Read the model definition and answer for the solid it produces. Units are mm, in the model's axes. A direction names the side the tool comes from. Coordinates: 2 decimals unless noted, no trailing zeros. Loops run counter-clockwise (first coordinate to the right, second up) from the corner with the lowest first, then second, coordinate; pieces in that order, holes last.
from build123d import *

# Parameters (mm, degrees)
SKETCH1_W                      = 120
SKETCH1_H                      = 200
BASE_FLANGE1_DEPTH             = 1.2
EDGE_FLANGE1_STRIP_W           = 6.2732
EDGE_FLANGE1_STRIP_H           = 1.2
EDGE_FLANGE1_STRIP_CUT_DEPTH   = 120
EDGE_FLANGE1_STRIP_2_W         = 6.2732
EDGE_FLANGE1_STRIP_2_H         = 1.2
EDGE_FLANGE1_STRIP_CUT_2_DEPTH = 120
EDGE_FLANGE1_DEPTH             = 120
EDGE_FLANGE1_BEND_DEPTH        = 120
EDGE_FLANGE3_START             = -121.9366
EDGE_FLANGE3_OUTLINE_W         = 50
EDGE_FLANGE3_OUTLINE_H         = 1.2
EDGE_FLANGE3_DEPTH             = 123.8732
EDGE_FLANGE3_START_2           = -25
EDGE_FLANGE3_2_DEPTH           = 50
EDGE_FLANGE3_START_3           = -65
EDGE_FLANGE3_3_DEPTH           = 130
EDGE_FLANGE4_STRIP_W           = 6.2732
EDGE_FLANGE4_STRIP_H           = 1.2
EDGE_FLANGE4_STRIP_CUT_DEPTH   = 120
EDGE_FLANGE4_STRIP_2_W         = 6.2732
EDGE_FLANGE4_STRIP_2_H         = 1.2
EDGE_FLANGE4_STRIP_CUT_2_DEPTH = 120
EDGE_FLANGE4_DEPTH             = 120
EDGE_FLANGE4_BEND_DEPTH        = 120
SKETCH34_R                     = 4
CUT_EXTRUDE1_DEPTH             = 10
CUT_EXTRUDE2_DEPTH             = 10
SKETCH36_R                     = 2.5
CUT_EXTRUDE3_DEPTH             = 243.320330787
SKETCH37_R                     = 2.5
CUT_EXTRUDE4_DEPTH             = 10


with BuildPart() as part:
    # Base-Flange1: sheet metal written as solids
    # Sketch1 → Base-Flange1 (new body)
    with BuildSketch(Plane.XY):
        Rectangle(SKETCH1_W, SKETCH1_H)
    extrude(amount=-BASE_FLANGE1_DEPTH)

    # Edge-Flange1: sheet metal written as solids
    # Edge-Flange1 strip (on a plane across the edge) → Edge-Flange1 strip cut (cut)
    with BuildSketch(Plane(origin=(-60, 100, -1.2), x_dir=(0, -1, 0), z_dir=(1, 0, 0))):
        with Locations((-1.2, -0.6)):
            Rectangle(EDGE_FLANGE1_STRIP_W, EDGE_FLANGE1_STRIP_H)
    extrude(amount=EDGE_FLANGE1_STRIP_CUT_DEPTH, mode=Mode.SUBTRACT)

    # Edge-Flange1 strip 2 (on a plane across the edge) → Edge-Flange1 strip cut 2 (cut)
    with BuildSketch(Plane(origin=(60, -100, -1.2), x_dir=(0, 1, 0), z_dir=(-1, 0, 0))):
        with Locations((-1.2, -0.6)):
            Rectangle(EDGE_FLANGE1_STRIP_2_W, EDGE_FLANGE1_STRIP_2_H)
    extrude(amount=EDGE_FLANGE1_STRIP_CUT_2_DEPTH, mode=Mode.SUBTRACT)

    # Edge-Flange1 section (on a plane across the edge) → Edge-Flange1 (add)
    with BuildSketch(Plane(origin=(-60, 100, -1.2), x_dir=(0, -1, 0), z_dir=(1, 0, 0))):
        with BuildLine():
            Line((0, 0.7366), (0, 178.8))
            Line((0, 178.8), (1.2, 178.8))
            Line((1.2, 178.8), (1.2, 0.7366))
            ThreePointArc((1.2, 0.7366), (1.415745145, 0.215745145), (1.9366, 0))
            Line((1.9366, 0), (1.9366, -1.2))
            ThreePointArc((1.9366, -1.2), (0.567217008, -0.632782992), (0, 0.7366))
        make_face()
    extrude(amount=EDGE_FLANGE1_DEPTH)

    # Edge-Flange1 section 2 (on a plane across the edge) → Edge-Flange1 bend (add)
    with BuildSketch(Plane(origin=(60, -100, -1.2), x_dir=(0, 1, 0), z_dir=(-1, 0, 0))):
        with BuildLine():
            Line((0, 0.7366), (0, 178.8))
            Line((0, 178.8), (1.2, 178.8))
            Line((1.2, 178.8), (1.2, 0.7366))
            ThreePointArc((1.2, 0.7366), (1.415745145, 0.215745145), (1.9366, 0))
            Line((1.9366, 0), (1.9366, -1.2))
            ThreePointArc((1.9366, -1.2), (0.567217008, -0.632782992), (0, 0.7366))
        make_face()
    extrude(amount=EDGE_FLANGE1_BEND_DEPTH)

    # Edge-Flange3: read off the stored shape, not the designer's step
    # Edge-Flange3 outline → Edge-Flange3 (add)
    with BuildSketch(Plane(origin=(60, 0, -1.2), x_dir=(0, -1, 0), z_dir=(1, 0, 0)).offset(EDGE_FLANGE3_START)):
        with Locations((0, -0.6)):
            Rectangle(EDGE_FLANGE3_OUTLINE_W, EDGE_FLANGE3_OUTLINE_H)
    extrude(amount=EDGE_FLANGE3_DEPTH)

    # Edge-Flange3 2 outline → Edge-Flange3 2 (add)
    with BuildSketch(Plane(origin=(0, 0, 0), x_dir=(1, 0, 0), z_dir=(0, 1, 0)).offset(EDGE_FLANGE3_START_2)):
        with BuildLine():
            ThreePointArc((61.9366, 0), (63.305982992, 0.567217008), (63.8732, 1.9366))
            Line((63.8732, 1.9366), (63.8732, 31.2))
            Line((63.8732, 31.2), (62.6732, 31.2))
            Line((62.6732, 31.2), (62.6732, 1.9366))
            ThreePointArc((62.6732, 1.9366), (62.457454855, 1.415745145), (61.9366, 1.2))
            Line((61.9366, 1.2), (61.9366, 0))
        make_face()
        with BuildLine():
            Line((-62.6732, 31.2), (-63.8732, 31.2))
            Line((-63.8732, 31.2), (-63.8732, 1.9366))
            ThreePointArc((-63.8732, 1.9366), (-63.305982992, 0.567217008), (-61.9366, 0))
            Line((-61.9366, 0), (-61.9366, 1.2))
            ThreePointArc((-61.9366, 1.2), (-62.457454855, 1.415745145), (-62.6732, 1.9366))
            Line((-62.6732, 1.9366), (-62.6732, 31.2))
        make_face()
    extrude(amount=EDGE_FLANGE3_2_DEPTH)

    # Edge-Flange3 3 outline → Edge-Flange3 3 (cut)
    with BuildSketch(Plane.YZ.offset(EDGE_FLANGE3_START_3)):
        with BuildLine():
            Line((-25, -31.2), (-15, -31.2))
            ThreePointArc((-15, -31.2), (-22.071067812, -28.271067812), (-25, -21.2))
            Line((-25, -21.2), (-25, -31.2))
        make_face()
        with BuildLine():
            ThreePointArc((25, -21.2), (22.071067812, -28.271067812), (15, -31.2))
            Line((15, -31.2), (25, -31.2))
            Line((25, -31.2), (25, -21.2))
        make_face()
    extrude(amount=EDGE_FLANGE3_3_DEPTH, mode=Mode.SUBTRACT)

    # Edge-Flange4: sheet metal written as solids
    # Edge-Flange4 strip (on a plane across the edge) → Edge-Flange4 strip cut (cut)
    with BuildSketch(Plane(origin=(-60, 98.8, -180), x_dir=(0, 0, 1), z_dir=(1, 0, 0))):
        with Locations((-1.2, -0.6)):
            Rectangle(EDGE_FLANGE4_STRIP_W, EDGE_FLANGE4_STRIP_H)
    extrude(amount=EDGE_FLANGE4_STRIP_CUT_DEPTH, mode=Mode.SUBTRACT)

    # Edge-Flange4 strip 2 (on a plane across the edge) → Edge-Flange4 strip cut 2 (cut)
    with BuildSketch(Plane(origin=(60, -98.8, -180), x_dir=(0, 0, 1), z_dir=(-1, 0, 0))):
        with Locations((-1.2, -0.6)):
            Rectangle(EDGE_FLANGE4_STRIP_2_W, EDGE_FLANGE4_STRIP_2_H)
    extrude(amount=EDGE_FLANGE4_STRIP_CUT_2_DEPTH, mode=Mode.SUBTRACT)

    # Edge-Flange4 section (on a plane across the edge) → Edge-Flange4 (add)
    with BuildSketch(Plane(origin=(-60, 98.8, -180), x_dir=(0, 0, 1), z_dir=(1, 0, 0))):
        with BuildLine():
            Line((0, 0.7366), (0, 18.8))
            Line((0, 18.8), (1.2, 18.8))
            Line((1.2, 18.8), (1.2, 0.7366))
            ThreePointArc((1.2, 0.7366), (1.415745145, 0.215745145), (1.9366, 0))
            Line((1.9366, 0), (1.9366, -1.2))
            ThreePointArc((1.9366, -1.2), (0.567217008, -0.632782992), (0, 0.7366))
        make_face()
    extrude(amount=EDGE_FLANGE4_DEPTH)

    # Edge-Flange4 section 2 (on a plane across the edge) → Edge-Flange4 bend (add)
    with BuildSketch(Plane(origin=(60, -98.8, -180), x_dir=(0, 0, 1), z_dir=(-1, 0, 0))):
        with BuildLine():
            Line((0, 0.7366), (0, 18.8))
            Line((0, 18.8), (1.2, 18.8))
            Line((1.2, 18.8), (1.2, 0.7366))
            ThreePointArc((1.2, 0.7366), (1.415745145, 0.215745145), (1.9366, 0))
            Line((1.9366, 0), (1.9366, -1.2))
            ThreePointArc((1.9366, -1.2), (0.567217008, -0.632782992), (0, 0.7366))
        make_face()
    extrude(amount=EDGE_FLANGE4_BEND_DEPTH)

    # Sketch34 → Cut-Extrude1 (cut)
    with BuildSketch(Plane.XZ.offset(100)):
        with Locations(Location((0, -90, 0), (0, 0, 270))):
            Circle(SKETCH34_R)
    extrude(amount=-CUT_EXTRUDE1_DEPTH, mode=Mode.SUBTRACT)

    # Sketch35 → Cut-Extrude2 (cut)
    with BuildSketch(Plane.XY):
        with BuildLine():
            Line((-31.3, -68), (-38.15, -68))
            ThreePointArc((-38.15, -68), (-39.564213562, -67.414213562), (-40.15, -66))
            Line((-40.15, -66), (-40.15, -54.035786438))
            Line((-40.15, -54.035786438), (-35.414213562, -49.3))
            Line((-35.414213562, -49.3), (-18.185786438, -49.3))
            Line((-18.185786438, -49.3), (-13.45, -54.035786438))
            Line((-13.45, -54.035786438), (-13.45, -66))
            ThreePointArc((-13.45, -66), (-14.035786438, -67.414213562), (-15.45, -68))
            Line((-15.45, -68), (-22.3, -68))
            Line((-22.3, -68), (-22.55, -68))
            Line((-22.55, -68), (-31.05, -68))
            Line((-31.05, -68), (-31.3, -68))
        make_face()
    extrude(amount=-CUT_EXTRUDE2_DEPTH, mode=Mode.SUBTRACT)

    # Sketch36 → Cut-Extrude3 (cut, through all)
    with BuildSketch(Plane.ZY.offset(63.8732)):
        with Locations((-15.6, 0)):
            Circle(SKETCH36_R)
    extrude(amount=-CUT_EXTRUDE3_DEPTH, mode=Mode.SUBTRACT)

    # Sketch37 → Cut-Extrude4 (cut)
    with BuildSketch(Plane(origin=(0, 0, -180), x_dir=(-1, 0, 0), z_dir=(0, 0, -1))):
        with Locations(Location((-30, 89.0317, 0), (0, 0, 90))):
            Circle(SKETCH37_R)
        with Locations(Location((30, 89.0317, 0), (0, 0, 90))):
            Circle(SKETCH37_R)
        with Locations(Location((30, -89.0317, 0), (0, 0, 90))):
            Circle(SKETCH37_R)
        with Locations(Location((-30, -89.0317, 0), (0, 0, 180))):
            Circle(SKETCH37_R)
    extrude(amount=-CUT_EXTRUDE4_DEPTH, mode=Mode.SUBTRACT)


solid = part.part
Q1. A cutting plane is placed at B-B (x = 30). Give the vertices of the cut face in (y, z).
Findings below:
outline: (-100, -178.06) arc R1.94 ccw to (-98.06, -180) - (-91.53, -180) - (-91.53, -178.8) - (-98.06, -178.8) arc R0.74 cw to (-98.8, -178.06) - (-98.8, -1.94) arc R0.74 cw to (-98.06, -1.2) - (98.06, -1.2) arc R0.74 cw to (98.8, -1.94) - (98.8, -178.06) arc R0.74 cw to (98.06, -178.8) - (91.53, -178.8) - (91.53, -180) - (98.06, -180) arc R1.94 ccw to (100, -178.06) - (100, -1.94) arc R1.94 ccw to (98.06, 0) - (-98.06, 0) arc R1.94 ccw to (-100, -1.94) - close; (-86.53, -180) - (-80, -180) - (-80, -178.8) - (-86.53, -178.8) - close; (80, -180) - (86.53, -180) - (86.53, -178.8) - (80, -178.8) - close
Q2. Straight lines are drawn through the part: probe 1 along Y at (x, z) = (-51, -122.5); probe 2 along Z at (x, y) = (19, -87); probe 3 along Z at (x, y) = (-36, 69.5). For each, find the intervals that lie inside material, in ascending order.
Findings below:
probe 1: y = -100 to -98.8, 98.8 to 100
probe 2: z = -180 to -178.8, -1.2 to 0
probe 3: z = -1.2 to 0
Q3. Determine the mould class of faces 6 (the face through (-63.873, 0, -20)), 7 (the face through (-1, 89, -178.8)), 8 (the face through (-1, 100, -89)) for opening direction Y: +Y half, -Y half, draft (parallel to the pull), parting line (faces both ways), or undercut.
Findings below:
face 6: draft
face 7: undercut
face 8: +Y half
Q4. Which of the six approach directions +Z, -Z, +X, -X, +Y, -Y give full straight-line access (tool end or side, diameter ignored) to faces 1 (the face through (29.67, -91.51, -179.41)), 2 (the face through (-62.673, 0, -20)), 3 (the face through (63.873, 0, -20)), 4 (the face through (-15.851, -51.635, -0.592)), 5 (the face through (1, -89, -178.8))?
Findings below:
face 1: -Z
face 2: -Z, +Y, -Y
face 3: +Z, -Z, +X, +Y, -Y
face 4: +Z, -Z
face 5: +X, -X
Q5. A cutting plane is placed at D-D (x = 0). Give the vertices of the cut face in (y, z).
Findings below:
outline: (-100, -178.06) arc R1.94 ccw to (-98.06, -180) - (-80, -180) - (-80, -178.8) - (-98.06, -178.8) arc R0.74 cw to (-98.8, -178.06) - (-98.8, -94) - (-100, -94) - close; (-100, -86) - (-98.8, -86) - (-98.8, -1.94) arc R0.74 cw to (-98.06, -1.2) - (98.06, -1.2) arc R0.74 cw to (98.8, -1.94) - (98.8, -178.06) arc R0.74 cw to (98.06, -178.8) - (80, -178.8) - (80, -180) - (98.06, -180) arc R1.94 ccw to (100, -178.06) - (100, -1.94) arc R1.94 ccw to (98.06, 0) - (-98.06, 0) arc R1.94 ccw to (-100, -1.94) - close
Q6. Flat-ended cylindrical pins translate along their axes: pin 1 Ø8 at (y, z) = (31, -24) entering from +X; pin 2 Ø0.6 at (x, y) = (63.5, 3) entering from -Z; pin 3 Ø3 at (x, y) = (45, 52.5) entering from -Z; pin 4 Ø0.6 at (y, z) = (-59.5, -0.5) entering from +X. Find the tip coordinate at first contact, or state that the pin passes through.
Findings below:
pin 1: passes through
pin 2: stops at z = -31.2
pin 3: stops at z = -1.2
pin 4: stops at x = 60
Q7. A cutting plane is placed at C-C (z = -153.5). Give the vertices of the cut face in (x, y), then the cut area to 3 significant figures.
Findings below:
outline: (-60, -100) - (60, -100) - (60, -98.8) - (-60, -98.8) - close; (-60, 98.8) - (60, 98.8) - (60, 100) - (-60, 100) - close
area: 288 mm2
Q8. A cutting plane is placed at A-A (x = -30). Count the separate pieces of the cut face and the enclosed holes in it, then the cut area to 3 significant figures.
Findings below:
separate pieces: 4
enclosed holes: 0
area: 677 mm2
